Geometry: final body of the model. Coordinates: model frame, mm. Coordinates: 2 decimals unless noted, no trailing zeros. Write each loop counter-clockwise with the first axis right and the second up, starting at its lowest first coordinate (ties: lowest second). Pieces come first, ordered by that corner, then holes. Notation, with made-up numbers: (56.5, 30.5) - (86.5, 30.5) arc R18 cw to (86.5, 43.5) - close; hole circle Ø11 at (-14, 10.25). An arc over 180 degrees is marked (long way). Put each result on its own line as item: value.
```python
from build123d import *

# Parameters (mm, degrees)
F0_W     = 0.7
F0_H     = 2
F2_SIZE2 = 0.2
F2_SIZE  = 0.2
F3_SIZE2 = 0.1
F3_SIZE  = 0.1
F4_SIZE2 = 0.2
F4_SIZE  = 0.2


# Not quite as in the source:
# - a fillet or chamfer that OpenCascade refuses, or shapes differently, is made with other operations: its cross-section is extruded or revolved along the edge and cut away or added


with BuildPart() as f1:
    # F0 (on Front) → F1 (revolve)
    with BuildSketch(Plane.XZ):
        Polygon((0, 38.25), (0, 36.75), (1, 36.75), (1, 38.25), (0.7, 38.25), align=None)
        Polygon((1, 36.75), (0, 36.75), (0, 0), (1, 0), (1.5, 0), (1.5, 17.425), (1.4, 17.525), (1.5, 17.625), (1.5, 17.925), (1.4, 18.025), (1.5, 18.125), (1.5, 18.425), (1.4, 18.525), (1.5, 18.625), (1.5, 19.125), (1.4, 19.225), (1.5, 19.325), (1.5, 36.75), align=None)
        with Locations((0.35, 39.25)):
            Rectangle(F0_W, F0_H)
        Polygon((1, 0), (0, 0), (0, -1.5), (0.7, -1.5), (1, -1.5), align=None)
        with Locations((0.35, -2.5)):
            Rectangle(F0_W, F0_H)
    revolve(axis=Axis((0, 0, 18.375), (0, 0, -1)))

    # F2
    f2_edges = [f1.edges().sort_by_distance(p)[0] for p in [
        (-0.7, 0, 40.25),
    ]]
    chamfer(f2_edges, length=F2_SIZE, length2=F2_SIZE2)

    # F3
    f3_edges = [f1.edges().sort_by_distance(p)[0] for p in [
        (-1.5, 0, 36.75),
    ]]
    chamfer(f3_edges, length=F3_SIZE, length2=F3_SIZE2)

    # F4
    f4_edges = [f1.edges().sort_by_distance(p)[0] for p in [
        (-0.7, 0, -3.5),
    ]]
    chamfer(f4_edges, length=F4_SIZE, length2=F4_SIZE2)

    # F5: chamfer of 0.1 on 2 edges, made by hand

    # F5_s1 → F5_t2 (revolve, cut)
    with BuildSketch(Plane.XZ):
        Polygon((1.4, 0), (1.5, 0.1), (1.5, 0), align=None)
    revolve(axis=Axis((0, 0, 0), (0, 0, -1)), mode=Mode.SUBTRACT)

    # F5_s3 → F5_t4 (revolve, cut)
    with BuildSketch(Plane.XZ):
        Polygon((1.4707106781, 19.2957106781), (1.5, 19.3664213562), (1.5, 19.325), align=None)
    revolve(axis=Axis((0, 0, 19.325), (0, 0, -1)), mode=Mode.SUBTRACT)


solid = f1.part
```
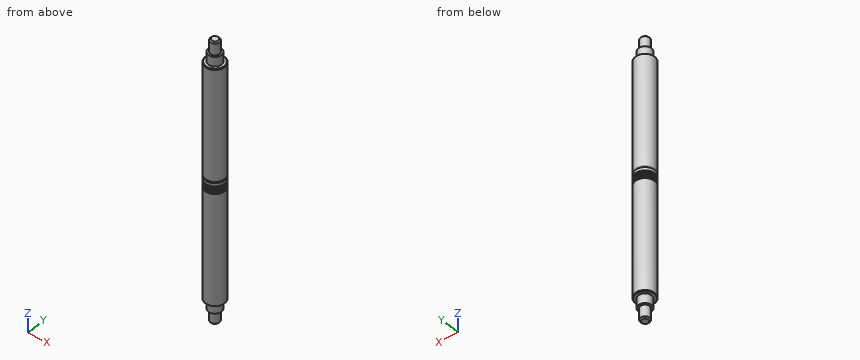
1. Ray query, probe 1 along Z at (x, y) = (-0.45, 0.6); probe 2 along Z at (x, y) = (1.1, 0.25); probe 3 along Y at (x, z) = (-0.55, 28). Return the intervals inside material, ascending. Write a range as from..to.
Answer below:
probe 1: z = -1.5..38.25
probe 2: z = 0..36.75
probe 3: y = -1.4..1.4
2. Pin query (flat end, axial travel): pin 1 Ø1 at (x, z) = (0.5, 26.5) entering from -Y. Return the tip coordinate at first contact, or that it passes through.
Answer below:
pin 1: stops at y = -1.5
3. Section query A-A (z = 7.5). Return loops of the section in (x, y).
Answer below:
outline: circle Ø3 at (0, 0)
